Design review of the part built by this model. Coordinates are the model's own, in mm. Face numbers are marked on the shaded views. A direction names the side the tool comes from. Coordinates: 2 decimals unless noted, no trailing zeros. Order: outer loops, then holes, each group sorted by start corner. A loop starts at its lowest first (then second) coordinate and runs counter-clockwise, first axis right, second up. Notation, with made-up numbers: (4.5, 66.25) -> (60.5, 66.25) arc R20 cw to (60.5, 82.25) -> close; hole circle Ø6 at (-1, 80.5). An arc over 180 degrees is marked (long way). Use a Markdown table: item, result. Add a question column.
Q1. Machinability: for the marked faces 1, 2, 3, 4 and 5, which of the approach directions +Z, -Z, +X, -X, +Y, -Y give a long, thin tool a straight path to every point of the face, cutting with its end or side? Answer none if there is none.
Q2. Add section C-C (z = 3.75). State the section outline as (x, y) points (3 decimals), then the cut area to 3 significant figures.
Q3. Add section A-A (y = -4). State the section outline as (x, z) points, then the cut area to 3 significant figures.
Q4. Wall thickness on probe 1 along Z at (x, y) = (2.55, 3.75); probe 2 along Y at (x, z) = (2.2, -8.5) (3 decimals); probe 3 along Z at (x, y) = (0.2, -4.5): over which ranges is each line inside the solid? List them lowest first.
Q5. Add section B-B (y = 0.25). State the section outline as (x, z) points, then the cut area to 3 significant figures.
Q6. The part is to be moulded in two halves that separate along Y. For the marked faces 6, 7, 8 and 9, say which applies: pulls with the +Y half, pulls with the -Y half, needs draft (parallel to the pull), parting line crosses it, or undercut.
Q7. Add section D-D (x = 1.7). State the section outline as (y, z) points (3 decimals).
Q8. Insertion check: pin 1 (2.5 mm diameter, centred on y = -4, z = 8.5, fed in from +X); pin 2 (2 mm diameter, centred on x = 3, z = 4, fed in from -Y); pin 3 (1.5 mm diameter, centred on x = 2, z = -7, fed in from -Y); pin 4 (1.1 mm diameter, centred on x = 1, z = 8.5, fed in from -Y). Each pin has a flat end and moves straight along its axis. Give the tip position at first contact, or say it passes through.
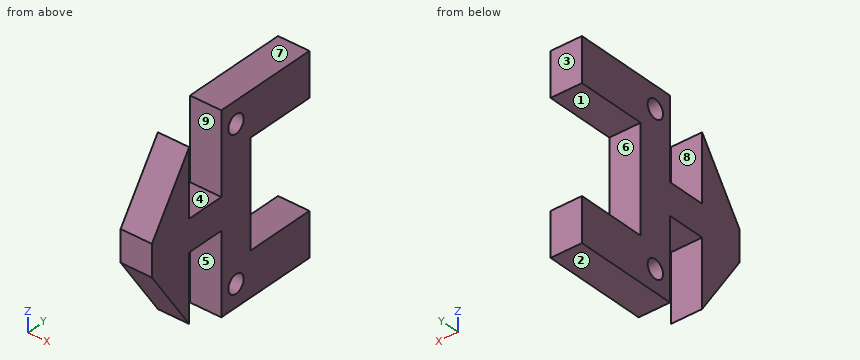
from build123d import *

# Parameters (mm, degrees)
BOSS_EXTRUDE1_DEPTH = 3.5814
SKETCH7_R           = 1.05
CUT_EXTRUDE5_DEPTH  = 14.03174685
BOSS_EXTRUDE3_DEPTH = 3.5814


with BuildPart() as part:
    # Sketch1 → Boss-Extrude1 (new body)
    with BuildSketch(Plane(origin=(0, 0, 0), x_dir=(0, 0, -1), z_dir=(1, 0, 0))):
        Polygon((-6, 6), (-6, -2), (6, -2), (6, 6), (11, 6), (11, -6), (-11, -6), (-11, 6), align=None)
    extrude(amount=BOSS_EXTRUDE1_DEPTH)

    # Sketch7 → Cut-Extrude5 (cut, through all)
    with BuildSketch(Plane(origin=(3.5814, 0, 0), x_dir=(0, 0, -1), z_dir=(1, 0, 0))):
        with Locations((-8.5, -4)):
            Circle(SKETCH7_R)
        with Locations((8.5, -4)):
            Circle(SKETCH7_R)
    extrude(amount=-CUT_EXTRUDE5_DEPTH, mode=Mode.SUBTRACT)

    # Sketch8 → Boss-Extrude3 (add)
    with BuildSketch(Plane(origin=(0, 0, 0), x_dir=(0, 0, -1), z_dir=(1, 0, 0))):
        Polygon((-1.7907, -10.3749976), (-9.398, -10.3749976), (-1.7907, -15.4549976), (1.7907, -15.4549976), (9.398, -10.3749976), (1.7907, -10.3749976), (1.7907, -6), (-1.7907, -6), align=None)
    extrude(amount=BOSS_EXTRUDE3_DEPTH)


solid = part.part
Established:
| question | item | result |
|---|---|---|
| 1 | face 1 | +X, -X, +Y |
| 1 | face 2 | -Z, +X, -X, +Y, -Y |
| 1 | face 3 | +Z, -Z, +X, -X, +Y |
| 1 | face 4 | +Z, +X, -X |
| 1 | face 5 | -Z, +X, -X |
| 2 | outline | (0, -14.147) -> (3.581, -14.147) -> (3.581, -10.375) -> (0, -10.375) -> close; (0, -6) -> (3.581, -6) -> (3.581, -2) -> (0, -2) -> close |
| 2 | area | 27.8 mm^2 |
| 3 | outline | (0, -11) -> (3.58, -11) -> (3.58, -9.55) -> (0, -9.55) -> close; (0, -7.45) -> (3.58, -7.45) -> (3.58, 7.45) -> (0, 7.45) -> close; (0, 9.55) -> (3.58, 9.55) -> (3.58, 11) -> (0, 11) -> close |
| 3 | area | 63.7 mm^2 |
| 4 | probe 1 | -11 to -6, 6 to 11 |
| 4 | probe 2 | -10.975 to -10.375, -6 to -5.05, -2.95 to 6 |
| 4 | probe 3 | -11 to -9.42, -7.58 to 7.58, 9.42 to 11 |
| 5 | outline | (0, -11) -> (3.58, -11) -> (3.58, -6) -> (0, -6) -> close; (0, 6) -> (3.58, 6) -> (3.58, 11) -> (0, 11) -> close |
| 5 | area | 35.8 mm^2 |
| 6 | face 6 | pulls with the +Y half |
| 6 | face 7 | needs draft |
| 6 | face 8 | undercut |
| 6 | face 9 | undercut |
| 7 | outline | (-15.455, -1.791) -> (-10.375, -9.398) -> (-10.375, -1.791) -> (-6, -1.791) -> (-6, -11) -> (6, -11) -> (6, -6) -> (-2, -6) -> (-2, 6) -> (6, 6) -> (6, 11) -> (-6, 11) -> (-6, 1.791) -> (-10.375, 1.791) -> (-10.375, 9.398) -> (-15.455, 1.791) -> close; hole circle Ø2.1 at (-4, -8.5); hole circle Ø2.1 at (-4, 8.5) |
| 8 | pin 1 | x = 3.58 |
| 8 | pin 2 | y = -14.65 |
| 8 | pin 3 | y = -12.48 |
| 8 | pin 4 | y = -11.34 |
